from build123d import *

# Parameters (mm, degrees)
SKETCH1_W              = 59.960812413
SKETCH1_H              = 103.12305947
SKETCH1_R              = 14.2875
BOSS_EXTRUDE1_DEPTH    = 3.175
CHAMFER1_SIZE          = 6.35
F_10_CLEARANCE_HOLE1_D = 5.6134


with BuildPart() as part:
    # Sketch1 → Boss-Extrude1 (new body)
    with BuildSketch(Plane.XY):
        with Locations((293.869593794, 80.109690656)):
            Rectangle(SKETCH1_W, SKETCH1_H)
        with Locations((293.869593793, 108.878190342)):
            Circle(SKETCH1_R, mode=Mode.SUBTRACT)
    extrude(amount=BOSS_EXTRUDE1_DEPTH)

    # Chamfer1
    chamfer1_edges = [part.edges().sort_by_distance(p)[0] for p in [
        (323.85, 28.548160921, 1.5875),
        (263.889187587, 28.548160921, 1.5875),
        (263.889187587, 131.671220391, 1.5875),
        (323.85, 131.671220391, 1.5875),
    ]]
    chamfer(chamfer1_edges, length=CHAMFER1_SIZE)

    # #10 Clearance Hole1 (through all)
    with Locations(Plane(origin=(0, 0, 0), x_dir=(1, 0, 0), z_dir=(0, 0, -1))):
        with Locations((275.136823716, -83.363402248), (275.136823716, -60.793377217), (313.56584092, -58.826399941), (313.56584092, -81.885554343), (275.136823716, -41.847646884), (313.56584092, -37.78667564)):
            Hole(F_10_CLEARANCE_HOLE1_D / 2)


solid = part.part
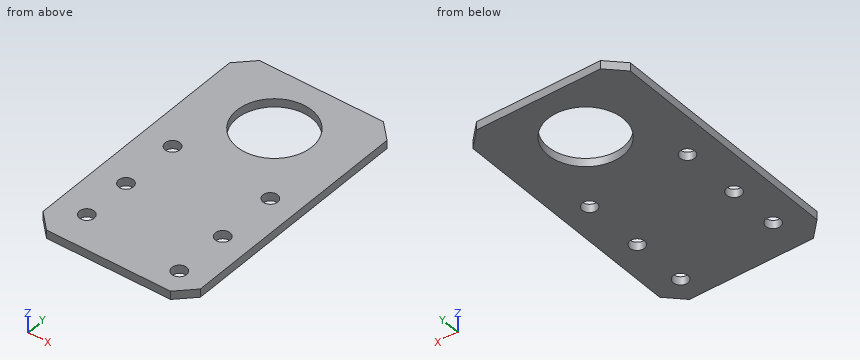
Could you check a few things on this model? Use its own coordinates, in mm. Give positions to 0.01 mm unless a question says otherwise; leave off trailing zeros. Order: outer loops, then holes, each group sorted by start corner. A loop starts at its lowest first (then second) coordinate and runs counter-clockwise, first axis right, second up.
1. I need wall thicknesses on L1, parallel to Y at x = 293.5, z = 0.5; L2, parallel to X at y = 111, z = 0.5; L3, parallel to X at y = 96, z = 1.7. Which ranges of each line are inside material? Lowest first, please.
2. Suppose I cut it at C-C (y = 100.5). List the corners of the cut face in (x, z) for me (3 decimals), plus the area to 3 significant figures.
3. Suppose I cut it at A-A (x = 284.5). List the corners of the cut face in (y, z) for me (3 decimals).
4. Suppose I cut it at B-B (z = 1.65). Give the number of separate pieces and of enclosed holes in the cut face, plus the area to 3 significant figures.
5. Suppose I cut it at D-D (x = 320.5). List the corners of the cut face in (y, z) for me (3 decimals).
Solved:
1. L1: y = 28.55 to 94.6, 123.16 to 131.67
1. L2: x = 263.89 to 279.74, 308 to 323.85
1. L3: x = 263.89 to 287.68, 300.06 to 323.85
2. outline: (263.889, 0) - (282.296, 0) - (282.296, 3.175) - (263.889, 3.175) - close; (305.443, 0) - (323.85, 0) - (323.85, 3.175) - (305.443, 3.175) - close
2. area: 117 mm2
3. outline: (28.548, 0) - (98.092, 0) - (98.092, 3.175) - (28.548, 3.175) - close; (119.664, 0) - (131.671, 0) - (131.671, 3.175) - (119.664, 3.175) - close
4. separate pieces: 1
4. enclosed holes: 7
4. area: 5,310 mm2
5. outline: (31.548, 0) - (128.671, 0) - (128.671, 3.175) - (31.548, 3.175) - close
